Verification items for the finished model (mm, model axes). Round coordinates to 2 decimals unless told otherwise and drop trailing zeros. Loops run counter-clockwise (first coordinate to the right, second up) from the corner with the lowest first, then second, coordinate; pieces in that order, holes last. Notation, with made-up numbers: M 22.25,32.25 L 28.25,32.25 A30 cw 28.25,69.25 Z; hole C -25,2 d4. An arc over 180 degrees is marked long. Write item = value, one per line. Start each with the question number.
from build123d import *

# Parameters (mm, degrees)
F0_W     = 350
F0_H     = 590
F1_DEPTH = 18
F3_DEPTH = 452


with BuildPart() as f1:
    # F0 (on Front) → F1 (new body)
    with BuildSketch(Plane.XZ):
        with Locations((175, 295)):
            Rectangle(F0_W, F0_H)
    extrude(amount=-F1_DEPTH)

    # F2 (on face) → F3 (cut)
    with BuildSketch(Plane(origin=(0, 0, 0), x_dir=(0, -1, 0), z_dir=(-1, 0, 0))):
        with BuildLine():
            Line((-5, 550), (0, 550))
            Line((0, 550), (0, 579))
            ThreePointArc((0, 579), (-5, 584), (-10, 579))
            Line((-10, 579), (-10, 555))
            ThreePointArc((-10, 555), (-8.535534, 551.464466), (-5, 550))
        make_face()
    extrude(amount=-F3_DEPTH, mode=Mode.SUBTRACT)


solid = f1.part
1. Mould release check, pull along Z, two halves, no side actions. Record for faces 1 (the flat face through (173, 0, 279)), 2 (the flat face through (173, 10, 567)), 3 (the flat face through (173, 9, 590)), 4 (the flat face through (173, 9, 0)): pulls with the +Z half, pulls with the -Z half, needs draft (parallel to the pull), parting line crosses it, or undercut.
2. Section check A-A, the plane x = 168. Enter the section's corners in (y, z), and give its area (3 significant figures).
3. Thickness scan on line 1 (Z direction, x = 89.5, y = 5.5); line 2 (Z direction, x = 181.5, y = 2). Record the ranges inside material, lowest first.
Computed values:
q1.face_1 = needs draft
q1.face_2 = undercut
q1.face_3 = pulls with the +Z half
q1.face_4 = pulls with the -Z half
q2.outline = M 0,0 L 18,0 L 18,590 L 0,590 L 0,579 A5 cw 10,579 L 10,555 A5 cw 5,550 L 0,550 Z
q2.area = 10,300 mm2
q3.line_1 = 0 to 550.03, 583.97 to 590
q3.line_2 = 0 to 550, 583 to 590
